Autodesk Inventor part; units mm, degrees
ref_plane "YZ Plane" through (0, 0, 0) normal (1, 0, 0) x (0, 1, 0)
ref_plane "XZ Plane" through (0, 0, 0) normal (0, 1, 0) x (-1, 0, 0)
ref_plane "XY Plane" through (0, 0, 0) normal (0, 0, 1) x (1, 0, 0)
sketch "Sketch1" plane through (0, 0, 0) normal (0, 0, 1) x (1, 0, 0)
  line L0 (-12.5, 12.5) -> (12.5, 12.5)
  line L1 (12.5, 12.5) -> (12.5, -12.5)
  line L2 (12.5, -12.5) -> (-12.5, -12.5)
  line L3 (-12.5, -12.5) -> (-12.5, 12.5)
  line L4 (-12.5, 12.5) -> (12.5, -12.5) construction
  line L5 (12.5, 12.5) -> (-12.5, -12.5) construction
  point P0 (0, 0)
  dimension "d0" = 25
  dimension "d1" = 25
extrude "Extrusion1" add sketch "Sketch1" along normal blind 6
sketch "Sketch2" plane through (-12.5, 12.5, 0) normal (0, 1, 0) x (1, 0, 0)
  circle A0 centre (2.75, -3) radius 1.75
  circle A1 centre (22.25, -3) radius 1.75
  line L0 (25, -6) -> (0, -6)
  line L1 (0, 0) -> (0, -6)
  line L2 (25, 0) -> (25, -6)
  point P0 (12.5, 0)
  dimension "d4" = 3
  dimension "d5" = 3.5
  dimension "d6" = 3.5
  dimension "d7" = 2.75
  dimension "d8" = 2.75
extrude "Extrusion2" add sketch "Sketch2" along normal blind 6
properties part number "watercoolerpatch"
Model file for the job. Use its own axes, mm. A direction names the side the tool comes from. Round coordinates to 2 decimals unless told otherwise and drop trailing zeros. Order: outer loops, then holes, each group sorted by start corner. A loop starts at its lowest first (then second) coordinate and runs counter-clockwise, first axis right, second up. Notation, with made-up numbers: (-12, -26.5) -> (38, -26.5) arc R23 cw to (38, 11.5) -> close; hole circle Ø1 at (-24, 70.5). An arc over 180 degrees is marked (long way). Use one line per item in the form item = value.
Item 1: Cut at D-D, the plane x = -6.25. Write the cut outline in (y, z), and give its area (3 significant figures).
Returned:
outline = (-12.5, 0) -> (12.5, 0) -> (12.5, 6) -> (-12.5, 6) -> close
area = 150 mm^2
Item 2: Pull direction X, two halves, no side cores. Call faces 1 (the face through (0, 0, 6)), 2 (the face through (12.5, 0, 3)), 3 (the face through (-8.94, 15.46, 1.45)): released by +X, released by -X, zero draft, split by the parting line, or undercut.
Returned:
face_1 = zero draft
face_2 = released by +X
face_3 = undercut
Item 3: Cut at A-A, the plane z = 3. Write the cut outline in (x, y).
Returned:
outline = (-12.5, -12.5) -> (12.5, -12.5) -> (12.5, 12.5) -> (11.5, 12.5) -> (11.5, 18.5) -> (8, 18.5) -> (8, 12.5) -> (-8, 12.5) -> (-8, 18.5) -> (-11.5, 18.5) -> (-11.5, 12.5) -> (-12.5, 12.5) -> close
Item 4: Cut at B-B, the plane x = -9.75. Write the cut outline in (y, z), and give its area (3 significant figures).
Returned:
outline = (-12.5, 0) -> (12.5, 0) -> (12.5, 1.25) -> (18.5, 1.25) -> (18.5, 4.75) -> (12.5, 4.75) -> (12.5, 6) -> (-12.5, 6) -> close
area = 171 mm^2
Item 5: Tool access for faces 4 (the face through (10, 18.5, 3)), 5 (the face through (10.56, 15.46, 1.45)): list every direction of +Z, -Z, +X, -X, +Y, -Y with a clear straight run to the whole face (end or side of a thin tool).
Returned:
face_4 = +Z, -Z, +X, -X, +Y
face_5 = +Y
Item 6: Cut at C-C, the plane y = 16.5. Write the cut outline in (x, z), and give its area (3 significant figures).
Returned:
outline = circle Ø3.5 at (-9.75, 3); circle Ø3.5 at (9.75, 3)
area = 19.2 mm^2
Item 7: Drill centre line: line 1 (Y direction, x = 3, z = 2.8). Where is it in solid material? Low to high.
Returned:
line_1 = -12.5 to 12.5
Item 8: Flat gauge pin, fed straight in: pin 1 Ø1.8 at (x, z) = (5, 3) entering from +Y. Where does the tip first touch, or does it go through?
Returned:
pin_1 = 12.5
